from build123d import *

# Parameters (mm, degrees)
F1_DEPTH    = 3
F2_T1_DEPTH = 42.4243909264
F2_T3_DEPTH = 68.8811967359
F2_T5_DEPTH = 42.4243909264


# Not quite as in the source:
# - a fillet or chamfer that OpenCascade refuses, or shapes differently, is made with other operations: its cross-section is extruded or revolved along the edge and cut away or added


with BuildPart() as f1:
    # F0 (on Top) → F1 (new body)
    with BuildSketch(Plane.XY):
        Polygon((50.666670315, 47.8041956116), (7.5023034588, 47.8041956116), (-6.7788518712, 39.1329097454), (-6.7788518712, -21.6580425002), (-1.982757669, -30.5968765852), (7.8172552019, -30.5968765852), (7.8172552019, -64.9542560763), (14.8365469649, -67.9511922197), (43.3324268088, -67.9511922197), (50.3517185719, -64.9542560763), (50.3517185719, -30.5968765852), (60.1517314427, -30.5968765852), (64.9478256449, -21.6580425002), (64.9478256449, 39.1329097454), align=None)
    extrude(amount=F1_DEPTH)

    # F2: chamfer of 5 on 3 edges, made by hand

    # F2_s2 → F2_t1 (cut)
    with BuildSketch(Plane(origin=(41.0836527068, -24.9453275187, 0), x_dir=(0, 0, 1), z_dir=(-0.8547719975, 0.5190036919, 0))):
        Polygon((5, 67.1578767244), (0, 62.1578767244), (0, 67.1578767244), align=None)
    extrude(amount=F2_T1_DEPTH, mode=Mode.SUBTRACT)

    # F2_s4 → F2_t3 (cut)
    with BuildSketch(Plane.YZ.offset(-5.3561114811)):
        Polygon((47.8041956116, 5), (42.8041956116, 0), (47.8041956116, 0), align=None)
    extrude(amount=F2_T3_DEPTH, mode=Mode.SUBTRACT)

    # F2_s6 → F2_t5 (cut)
    with BuildSketch(Plane(origin=(37.6798265821, 22.8785795082, 0), x_dir=(0, 0, 1), z_dir=(-0.8547719975, -0.5190036919, 0))):
        Polygon((5, 36.9679645806), (0, 31.9679645806), (0, 36.9679645806), align=None)
    extrude(amount=F2_T5_DEPTH, mode=Mode.SUBTRACT)


solid = f1.part
Geometry: final body of the model. Coordinates: model frame, mm. A direction names the side the tool comes from. Round coordinates to 2 decimals unless told otherwise and drop trailing zeros. Loops run counter-clockwise (first coordinate to the right, second up) from the corner with the lowest first, then second, coordinate; pieces in that order, holes last. Notation, with made-up numbers: (46.5, -14.5) - (97.5, -14.5) arc R17 ccw to (97.5, 2.5) - close; hole circle Ø2 at (-35, -8). An arc over 180 degrees is marked (long way). Write each question's results on one line, items separated by ' | '. Start each with the question number.
1) Cut plane C-C on x = 59. Return loops of the section in (y, z).
2) First-contact query: P1, Ø8, axis at x = 45.5, y = 5, coming from the -Z side; P2, Ø0.9, axis at x = 56.5, z = 1.5, coming from the -Y side; P3, Ø1, axis at x = 5, z = 0.5, coming from the +Y side; P4, Ø0.9, axis at y = -48, z = 2, coming from the +X side. Flat tips, straight axial feed; report the tip coordinate or a pass-through.
3) Cut plane A-A on z = 1. Return loops of the section in (x, y).
4) Access query for faces 1 (the face through (0.75, 39.63, 1.52)), 2 (the face through (3, -30.597, 1)), 3 (the face through (55, -30.597, 1)). Directions: +Z, -Z, +X, -X, +Y, -Y. A direction counts if a zero-diameter tool reaches every point of the face in a straight line with its end or side. Return the directions, or none.
5) Line query: probe 1 along X at (y, z) = (-58, 1.75); probe 2 along Y at (x, z) = (60, 0.5); probe 3 along Y at (x, z) = (43, 2.8). Output: solid intervals per line, ascending. Write a range as [from, to].
6) Cut plane B-B on y = -42.5. Return loops of the section in (x, z), then the cut area to 3 significant figures.
Verdict:
1) outline: (-30.6, 0) - (36.89, 0) - (40.4, 3) - (-30.6, 3) - close
2) P1: stops at z = 0 | P2: stops at y = -30.6 | P3: stops at y = 41.68 | P4: stops at x = 50.35
3) outline: (-6.78, -21.66) - (-1.98, -30.6) - (7.82, -30.6) - (7.82, -64.95) - (14.84, -67.95) - (43.33, -67.95) - (50.35, -64.95) - (50.35, -30.6) - (60.15, -30.6) - (64.95, -21.66) - (64.95, 34.45) - (49.55, 43.8) - (8.62, 43.8) - (-6.78, 34.45) - close
4) face 1: -Z, -X, +Y | face 2: +Z, -Z, -X, -Y | face 3: +Z, -Z, +X, -Y
5) probe 1: x = [7.82, 50.35] | probe 2: y = [-30.6, 36.87] | probe 3: y = [-67.95, 45.6]
6) outline: (7.82, 0) - (50.35, 0) - (50.35, 3) - (7.82, 3) - close | area: 128 mm2
